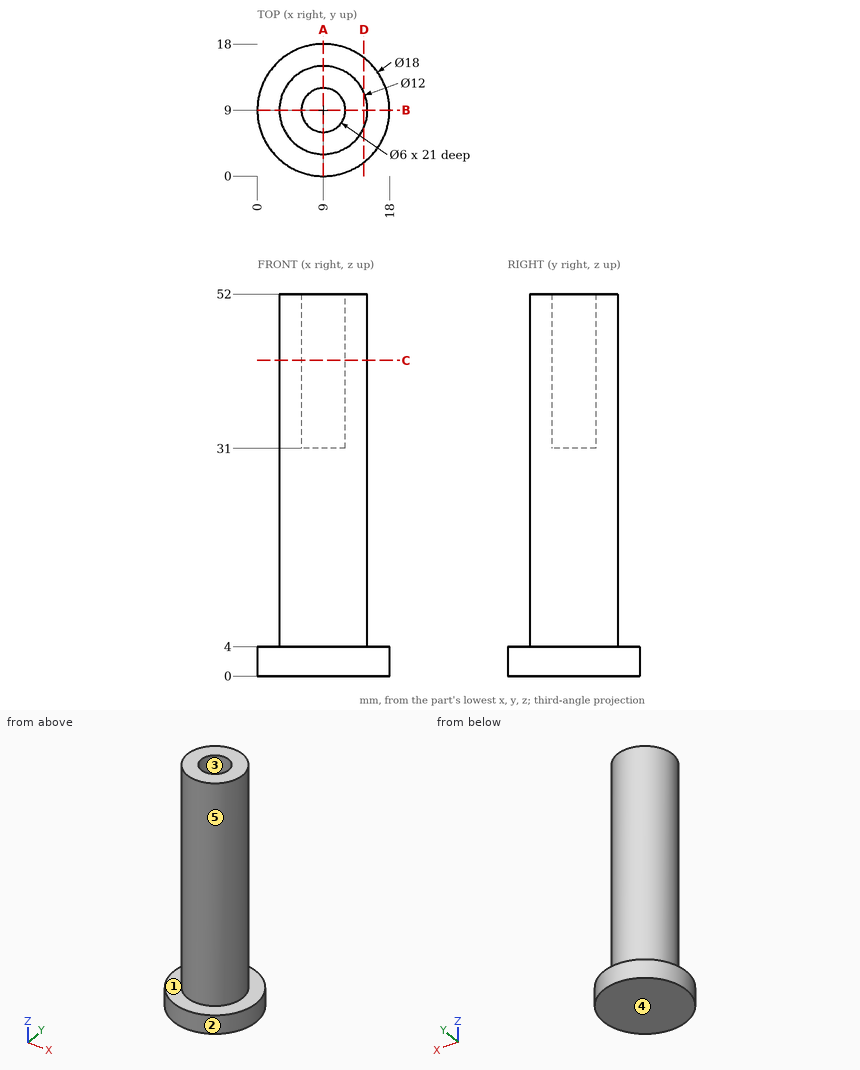
Design review of the part shown in the three views and the two pictorial views. Dimensions are in mm from the part's minimum x, y and z. A direction names the side the tool comes from. Coordinates: 2 decimals unless noted, no trailing zeros. Order: outer loops, then holes, each group sorted by start corner. A loop starts at its lowest first (then second) coordinate and runs counter-clockwise, first axis right, second up.
1) Wall thickness on line 1 along Y through (x, z) = (9, 36.25); line 2 along Y through (x, z) = (8.75, 6.5); line 3 along Z through (x, y) = (10, 11): over which ranges is each line inside the solid? List them lowest first.
2) Clearance check with flat-ended pins moving along their axes: pin 1 (5 mm diameter, centred on x = 13.5, z = 35.5, fed in from +Y); pin 2 (4 mm diameter, centred on y = 5, z = 6.5, fed in from -X); pin 3 (2 mm diameter, centred on y = 9.5, z = 18, fed in from +X); pin 4 (5 mm diameter, centred on x = 10, y = 8, fed in from +Z). State where each tip first meets the part, or that it passes through.
3) Take a section at D-D, the plane x = 14.5. Give the boundary of the cut face in (y, z), and give its area (3 significant figures).
4) For the marked faces 4 and 5, list the 3-axis set-ups (+Z, -Z, +X, -X, +Y, -Y) from which the entire face can be reached by the end or side of a thin tool; tool diameter is ignored.
5) Take a section at C-C, the plane z = 43. Give the boundary of the cut face in (x, y).
6) Take a section at A-A, the plane x = 9. Give the boundary of the cut face in (y, z), and give its area (3 significant figures).
7) Mouldability with a two-part tool opening along X and no side actions: class the marked faces 1, 2 and 3 as +X half, -X half, draft (parallel to the pull), parting line (faces both ways), or undercut.
Returned:
1. line 1: y = 3 to 6, 12 to 15
1. line 2: y = 3.01 to 14.99
1. line 3: z = 0 to 31
2. pin 1: stops at y = 14.66
2. pin 2: stops at x = 3.34
2. pin 3: stops at x = 15
2. pin 4: stops at z = 52
3. outline: (1.88, 0) - (16.12, 0) - (16.12, 4) - (11.4, 4) - (11.4, 52) - (6.6, 52) - (6.6, 4) - (1.88, 4) - close
3. area: 287 mm2
4. face 4: -Z, +X, -X, +Y, -Y
4. face 5: +Z
5. outline: circle Ø12 at (9, 9); hole circle Ø6 at (9, 9)
6. outline: (0, 0) - (18, 0) - (18, 4) - (15, 4) - (15, 52) - (12, 52) - (12, 31) - (6, 31) - (6, 52) - (3, 52) - (3, 4) - (0, 4) - close
6. area: 522 mm2
7. face 1: draft
7. face 2: parting line
7. face 3: undercut
